from build123d import *

# Parameters (mm, degrees)
SKETCH2_W                                      = 101.6
SKETCH2_H                                      = 76.2
BOSS_EXTRUDE1_DEPTH                            = 6.35
CBORE_FOR_4_SOCKET_HEAD_CAP_SCREW1_D           = 3.2639
CBORE_FOR_4_SOCKET_HEAD_CAP_SCREW1_CBORE_D     = 5.55752
CBORE_FOR_4_SOCKET_HEAD_CAP_SCREW1_CBORE_DEPTH = 2.8448
F_8_32_TAPPED_HOLE1_D                          = 3.4544


with BuildPart() as part:
    # Sketch2 → Boss-Extrude1 (new body)
    with BuildSketch(Plane(origin=(0, 0, 0), x_dir=(1, 0, 0), z_dir=(0, 1, 0))):
        Rectangle(SKETCH2_W, SKETCH2_H)
        with BuildLine():
            Line((-19.05, 33.02), (19.05, 33.02))
            ThreePointArc((19.05, 33.02), (23.540128061, 31.160128061), (25.4, 26.67))
            Line((25.4, 26.67), (25.4, -26.67))
            ThreePointArc((25.4, -26.67), (23.540128061, -31.160128061), (19.05, -33.02))
            Line((19.05, -33.02), (-19.05, -33.02))
            ThreePointArc((-19.05, -33.02), (-23.540128061, -31.160128061), (-25.4, -26.67))
            Line((-25.4, -26.67), (-25.4, 26.67))
            ThreePointArc((-25.4, 26.67), (-23.540128061, 31.160128061), (-19.05, 33.02))
        make_face(mode=Mode.SUBTRACT)
    extrude(amount=BOSS_EXTRUDE1_DEPTH)

    # CBORE for #4 Socket Head Cap Screw1 (through all)
    with Locations(Plane(origin=(0, 6.35, 0), x_dir=(1, 0, 0), z_dir=(0, 1, 0))):
        with Locations((-29.972, 29.972), (29.972, 29.972), (29.972, -29.972), (-29.972, -29.972)):
            CounterBoreHole(CBORE_FOR_4_SOCKET_HEAD_CAP_SCREW1_D / 2, CBORE_FOR_4_SOCKET_HEAD_CAP_SCREW1_CBORE_D / 2, CBORE_FOR_4_SOCKET_HEAD_CAP_SCREW1_CBORE_DEPTH)

    # #8-32 Tapped Hole1 (through all)
    with Locations(Plane(origin=(0, 6.35, 0), x_dir=(1, 0, 0), z_dir=(0, 1, 0))):
        with Locations((-45.339, 16.129), (-45.466, -21.971), (43.561, 16.129), (43.434, -21.971)):
            Hole(F_8_32_TAPPED_HOLE1_D / 2)


solid = part.part
Design review of the part built by this model. Coordinates are the model's own, in mm. A direction names the side the tool comes from. Round coordinates to 2 decimals unless told otherwise and drop trailing zeros. Write each loop counter-clockwise with the first axis right and the second up, starting at its lowest first coordinate (ties: lowest second). Pieces come first, ordered by that corner, then holes. Notation, with made-up numbers: (45.5, -8.5) - (73.5, -8.5) arc R23 cw to (73.5, 0.5) - close; hole circle Ø6 at (60.25, 70). An arc over 180 degrees is marked (long way). Use a Markdown table: item, result. Add a question column.
1. For faces 1 (the face through (-0.7, 0, 33.3)), 2 (the face through (27.924, 4.948, 28.094)), 3 (the face through (23.6, 3.1, 31.1)), list the 3-axis set-ups (+Z, -Z, +X, -X, +Y, -Y) from which the entire face can be reached by the end or side of a thin tool; tool diameter is ignored.
2. Wall thickness on probe 1 along X at (y, z) = (4.25, -20.5); probe 2 along Z at (x, y) = (1, 5.25); probe 3 along Z at (x, y) = (-44, 4.25): over which ranges is each line inside the solid? List them lowest first.
3. We need section A-A (z = -10.5). State the section outline as (x, y) points, then the cut area to 3 significant figures.
4. Mouldability with a two-part tool opening along Z and no side actions: class faces 4 (the face through (-1, 3, 38.1)), 5 (the face through (0, 3, 33.02)), 6 (the face through (-0.7, 6.35, 33.3)) as +Z half, -Z half, draft (parallel to the pull), parting line (faces both ways), or undercut.
5. We need section B-B (x = -3). State the section outline as (y, z) points, then the cut area to 3 significant figures.
6. We need section C-C (y = 4.75). Count the separate pieces of the cut face and the enclosed holes in it, then the cut area to 3 significant figures.
7. Clearance check with flat-ended pins moving along their axes: pin 1 (9 mm diameter, centred on x = -29.972, z = 29.972, fed in from +Y); pin 2 (1.7 mm diameter, centred on x = -29.5, z = 31, fed in from +Y); pin 3 (3 mm diameter, centred on x = 43.434, z = 21.971, fed in from -Y). State where each tip first meets the part, or that it passes through.
Output:
| question | item | result |
|---|---|---|
| 1 | face 1 | +Z, -Z, +X, -X, -Y |
| 1 | face 2 | +Y |
| 1 | face 3 | +Y, -Y |
| 2 | probe 1 | x = -50.8 to -25.4, 25.4 to 50.8 |
| 2 | probe 2 | z = -38.1 to -33.02, 33.02 to 38.1 |
| 2 | probe 3 | z = -38.1 to -17.22, -15.04 to 21.06, 22.88 to 38.1 |
| 3 | outline | (-50.8, 0) - (-25.4, 0) - (-25.4, 6.35) - (-50.8, 6.35) - close; (25.4, 0) - (50.8, 0) - (50.8, 6.35) - (25.4, 6.35) - close |
| 3 | area | 323 mm2 |
| 4 | face 4 | +Z half |
| 4 | face 5 | undercut |
| 4 | face 6 | draft |
| 5 | outline | (0, -38.1) - (6.35, -38.1) - (6.35, -33.02) - (0, -33.02) - close; (0, 33.02) - (6.35, 33.02) - (6.35, 38.1) - (0, 38.1) - close |
| 5 | area | 64.5 mm2 |
| 6 | separate pieces | 1 |
| 6 | enclosed holes | 9 |
| 6 | area | 4,290 mm2 |
| 7 | pin 1 | stops at y = 6.35 |
| 7 | pin 2 | stops at y = 3.51 |
| 7 | pin 3 | passes through |
